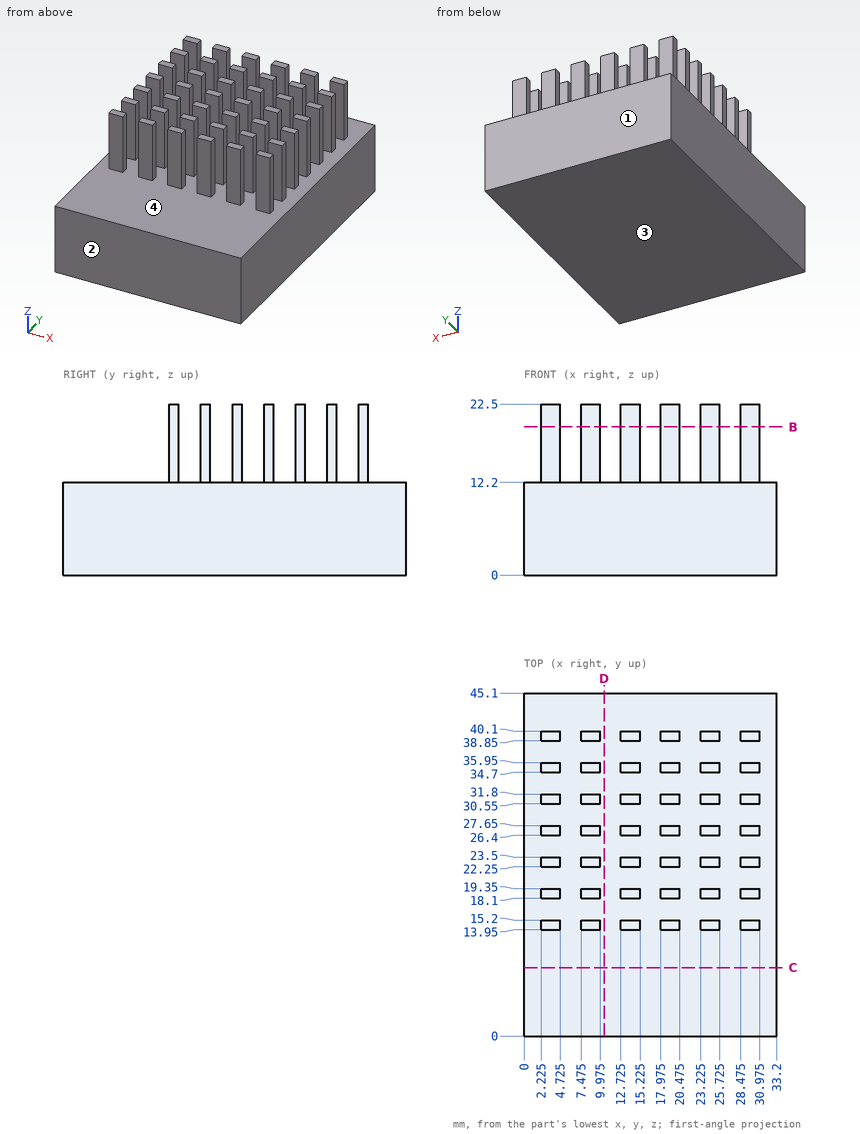
The figure shows three views and two pictorial views of one solid part (mm, origin at its lowest corner). Answer the questions. Round coordinates to 2 decimals unless told otherwise and drop trailing zeros. Write each loop counter-clockwise with the first axis right and the second up, starting at its lowest first coordinate (ties: lowest second). Pieces come first, ordered by that corner, then holes. Notation, with made-up numbers: (-16.75, -18.5) -> (20.25, -18.5) arc R11 cw to (20.25, -7.5) -> close; hole circle Ø1 at (79.25, -35.5). An arc over 180 degrees is marked (long way). Write each question's results on one line, items separated by ' | '.
Q1. Determine the mould class of the marked faces 1, 2, 3 and 4 for opening direction Y: released by +Y, released by -Y, zero draft, split by the parting line, or undercut.
Data:
face 1: released by +Y | face 2: released by -Y | face 3: zero draft | face 4: undercut
Q2. Straight lines are drawn through the part: line 1 along X through (y, z) = (23, 15.5) (3 decimals); line 2 along Z through (x, y) = (8, 8.5). For each, find the intervals that lie inside material, in ascending order. Write a range as [from, to].
Data:
line 1: [2.225, 4.725], [7.475, 9.975], [12.725, 15.225], [17.975, 20.475], [23.225, 25.725], [28.475, 30.975] | line 2: [0, 12.2]
Q3. Section D-D, the plane x = 10.5 is taken. Write down the section's boundary in (y, z), then the cut area to 3 significant figures.
Data:
outline: (0, 0) -> (45.1, 0) -> (45.1, 12.2) -> (0, 12.2) -> close | area: 550 mm^2
Q4. Section B-B, the plane z = 19.5 is taken. Give the number of separate pieces and of enclosed holes in the cut face, then the cut area to 3 significant figures.
Data:
separate pieces: 42 | enclosed holes: 0 | area: 131 mm^2
Q5. Section C-C, the plane y = 9 is taken. Write down the section's boundary in (x, z), then the cut area to 3 significant figures.
Data:
outline: (0, 0) -> (33.2, 0) -> (33.2, 12.2) -> (0, 12.2) -> close | area: 405 mm^2
Q6. Flat-ended cylindrical pins translate along their axes: P1, Ø2, axis at x = 18.5, z = 19, coming from the -Y side; P2, Ø0.8, axis at x = 9, z = 18.5, coming from the +Y side; P3, Ø1.4, axis at y = 35, z = 19.5, coming from the -X side (3 decimals); P4, Ø3, axis at x = 25.5, y = 24, coming from the +Z side. Find the tip coordinate at first contact, or state that the pin passes through.
Data:
P1: y = 13.95 | P2: y = 40.1 | P3: x = 2.225 | P4: z = 22.5
